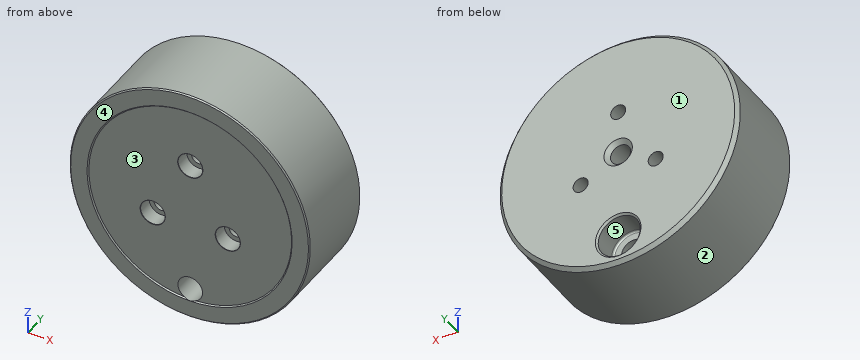
```python
from build123d import *

# Parameters (mm, degrees)
M10X1_5_TAPPED_HOLE1_D           = 8.5
M10X1_5_TAPPED_HOLE1_DEPTH       = 24.4856
M10X1_5_TAPPED_HOLE1_CSINK_D     = 12
M10X1_5_TAPPED_HOLE1_CSINK_ANGLE = 90
M10X1_5_TAPPED_HOLE1_TIP         = 2.553657631
HOLE1_D                          = 6.35
HOLE1_DEPTH                      = 37.592
HOLE1_CBORE_D                    = 10.414
HOLE1_CBORE_DEPTH                = 6.35
HOLE1_TIP                        = 1.907732465
CHAMFER1_SIZE                    = 1.524
CHAMFER2_SIZE                    = 0.762
CHAMFER3_SIZE                    = 0.508
CHAMFER4_SIZE                    = 0.127
FILLET1_R                        = 0.8128


with BuildPart() as part:
    # Sketch1 → Revolve1 (revolve)
    with BuildSketch(Plane.XY, mode=Mode.PRIVATE) as revolve1_sk:
        Polygon((0, 0.508), (42.8625, 0.508), (43.3705, 0), (50.8, 0), (50.8, 38.1), (0, 38.1), align=None)
    revolve(revolve1_sk.sketch.rotate(Axis((0, 0, 0), (0, 1, 0)), 90), axis=Axis((0, 0, 0), (0, 1, 0)))  # turned: the seam where the file's is

    # Sketch2 → Cut-Revolve1 (revolve, cut)
    with BuildSketch(Plane(origin=(0, 0, 0), x_dir=(0, 0, -1), z_dir=(1, 0, 0))):
        Polygon((38.1, 38.1), (46.99, 38.1), (46.99, 26.67), (43.307, 26.67), (43.307, 0), (38.1, 0), align=None)
    revolve(axis=Axis((0, 38.1, -38.1), (0, 1, 0)), mode=Mode.SUBTRACT)

    # M10x1.5 Tapped Hole1
    with Locations(Plane(origin=(0, 38.1, 0), x_dir=(-1, 0, 0), z_dir=(0, 1, 0))):
        with Locations((0, 0)):
            CounterSinkHole(M10X1_5_TAPPED_HOLE1_D / 2, M10X1_5_TAPPED_HOLE1_CSINK_D / 2, depth=M10X1_5_TAPPED_HOLE1_DEPTH, counter_sink_angle=M10X1_5_TAPPED_HOLE1_CSINK_ANGLE)
            with Locations((0, 0, -(M10X1_5_TAPPED_HOLE1_DEPTH + M10X1_5_TAPPED_HOLE1_TIP / 2))):  # 118° drill point
                Cone(0, M10X1_5_TAPPED_HOLE1_D / 2, M10X1_5_TAPPED_HOLE1_TIP, mode=Mode.SUBTRACT)

    # Hole1
    with Locations(Plane.XZ.offset(-0.508)):
        with Locations((0, 18.330871047), (15.875, -9.165435523), (-15.875, -9.165435523)):
            CounterBoreHole(HOLE1_D / 2, HOLE1_CBORE_D / 2, HOLE1_CBORE_DEPTH, depth=HOLE1_DEPTH)
            with Locations((0, 0, -(HOLE1_DEPTH + HOLE1_TIP / 2))):  # 118° drill point
                Cone(0, HOLE1_D / 2, HOLE1_TIP, mode=Mode.SUBTRACT)

    # Chamfer1
    chamfer1_edges = [part.edges().sort_by_distance(p)[0] for p in [
        (0, 38.1, 50.8),
    ]]
    chamfer(chamfer1_edges, length=CHAMFER1_SIZE)

    # Chamfer2
    chamfer2_edges = [part.edges().sort_by_distance(p)[0] for p in [
        (0, 38.1, -29.21),
    ]]
    chamfer(chamfer2_edges, length=CHAMFER2_SIZE)

    # Chamfer3
    chamfer3_edges = [part.edges().sort_by_distance(p)[0] for p in [
        (0, 0, 50.8),
    ]]
    chamfer(chamfer3_edges, length=CHAMFER3_SIZE)

    # Chamfer4
    chamfer4_edges = [part.edges().sort_by_distance(p)[0] for p in [
        (-21.082, 0.508, -9.165435523),
        (10.668, 0.508, -9.165435523),
        (-5.207, 0.508, 18.330871047),
    ]]
    chamfer(chamfer4_edges, length=CHAMFER4_SIZE)

    # Fillet1
    fillet1_edges = [part.edges().sort_by_distance(p)[0] for p in [
        (0, 26.67, -29.21),
    ]]
    fillet(fillet1_edges, radius=FILLET1_R)


solid = part.part
```
The listing builds one solid part. Answer for the finished solid, in the listing's coordinates (mm). Face numbers are marked on the shaded views. A direction names the side the tool comes from. Give positions to 0.01 mm unless a question says otherwise; leave off trailing zeros. Write each loop counter-clockwise with the first axis right and the second up, starting at its lowest first coordinate (ties: lowest second). Pieces come first, ordered by that corner, then holes. Notation, with made-up numbers: (20, -30) -> (40, -30) arc R23 ccw to (40, -15) -> close; hole circle Ø6 at (-34, -33.5). An arc over 180 degrees is marked (long way). Write item = value, one per line. Start each with the question number.
1) Which of the six approach directions +Z, -Z, +X, -X, +Y, -Y give full straight-line access (tool end or side, diameter ignored) to the marked faces 4 and 5?
2) Each of these flat-tipped pins is pushed along its axis until it touches: pin 1 (2 mm diameter, centred on x = -11.5, z = 35.5, fed in from -Y); pin 2 (9.5 mm diameter, centred on x = 0, z = -38.1, fed in from +Y); pin 3 (7 mm diameter, centred on x = 0, z = 0, fed in from +Y); pin 4 (12 mm diameter, centred on y = 26.5, z = -17, fed in from +X). Where does it stop, or does it pass through?
3) Straight lines are drawn through the part: line 1 along X through (y, z) = (35.5, -8); line 2 along Z through (x, y) = (1, 30); line 3 along Y through (x, z) = (-0.5, 11). For each, find the intervals that lie inside material, in ascending order.
4) The part is cut by section B-B, the plane y = 31.5. Determine the outline of the cut face in (x, z) (3 decimals), and give its area (3 significant figures).
5) The part is cut by section A-A, the plane y = 24. Determine the outline of the cut face in (x, z) (3 decimals).
6) Determine the mould class of the marked faces 1, 2 and 3 for opening direction X: +X half, -X half, draft (parallel to the pull), parting line (faces both ways), or undercut.
Solutions:
q1.face_4 = +Z, -Z, +X, -X, -Y
q1.face_5 = +Y
q2.pin_1 = 0.51
q2.pin_2 = through
q2.pin_3 = 13.16
q2.pin_4 = 49.59
q3.line_1 = -50.17 to -18.83, -12.92 to 12.92, 18.83 to 50.17
q3.line_2 = -50.79 to -46.93, -29.27 to -4.13, 4.13 to 15.32, 21.34 to 50.79
q3.line_3 = 0.51 to 38.1
q4.outline = circle Ø101.6 at (0, 0); hole circle Ø6.35 at (-15.875, -9.165); hole circle Ø17.78 at (0, -38.1); hole circle Ø8.5 at (0, 0); hole circle Ø6.35 at (0, 18.331); hole circle Ø6.35 at (15.875, -9.165)
q4.area = 7,710 mm²
q5.outline = circle Ø101.6 at (0, 0); hole circle Ø6.35 at (-15.875, -9.165); hole circle Ø10.414 at (0, -38.1); hole circle Ø8.5 at (0, 0); hole circle Ø6.35 at (0, 18.331); hole circle Ø6.35 at (15.875, -9.165)
q6.face_1 = draft
q6.face_2 = parting line
q6.face_3 = undercut
